The model under review builds one solid part; all positions refer to its coordinate system, in mm. Face numbers are marked on the shaded views. A direction names the side the tool comes from. Give positions to 0.01 mm unless a question says otherwise; leave off trailing zeros. Order: outer loops, then holes, each group sorted by start corner. A loop starts at its lowest first (then second) coordinate and runs counter-clockwise, first axis right, second up. Notation, with made-up numbers: (39, 5) - (71, 5) arc R6 ccw to (71, 9) - close; hole circle Ø6 at (41, 50.25). An arc over 180 degrees is marked (long way). Use CSV: the item, a comma, the result in double quotes.
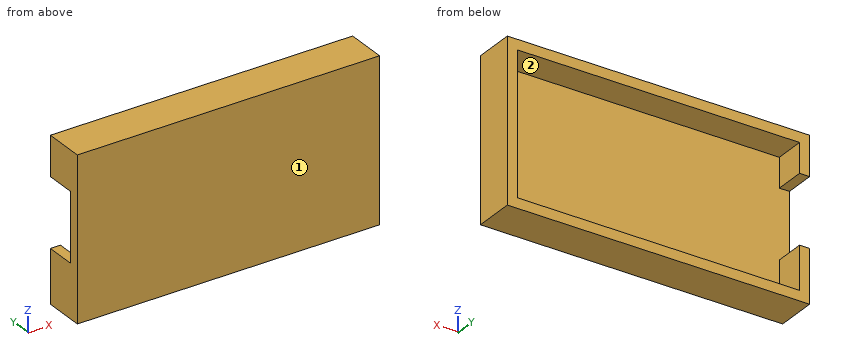
```python
from build123d import *

# Parameters (mm, degrees)
F0_W     = 2.5
F0_H     = 17
F1_DEPTH = 10
F2_DEPTH = 7.5


# Not quite as in the source:
# - a feature names something its author has since deleted; it is built from what else it names


with BuildPart() as f1:
    # F0 (on Front) → F1 (new body)
    with BuildSketch(Plane.XZ):
        Polygon((37.5, 20), (-37.5, 20), (-37.5, 10.2), (-35, 10.2), (-35, 17.5), (35, 17.5), (35, -17.5), (-35, -17.5), (-35, -6.8), (-37.5, -6.8), (-37.5, -20), (37.5, -20), align=None)
        with Locations((-36.25, 1.7)):
            Rectangle(F0_W, F0_H)
        Polygon((-35, 17.5), (-35, 10.2), (-35, -6.8), (-35, -17.5), (35, -17.5), (35, 17.5), align=None)
    extrude(amount=F1_DEPTH)

    # F0 (on Front) → F2 (cut)
    with BuildSketch(Plane.XZ):
        Polygon((-35, 17.5), (-35, 10.2), (-35, -6.8), (-35, -17.5), (35, -17.5), (35, 17.5), align=None)
        with Locations((-36.25, 1.7)):
            Rectangle(F0_W, F0_H)
    extrude(amount=F2_DEPTH, mode=Mode.SUBTRACT)


solid = f1.part
```
Item 1: Tool access review of the marked faces 1 and 2: name each direction out of +Z, -Z, +X, -X, +Y, -Y from which nothing blocks a thin tool from reaching the whole face with its end or side.
Results list:
face 1,"+Z, -Z, +X, -X, -Y"
face 2,"+Y"
Item 2: Take a section at A-A, the plane z = -12. Give the boundary of the cut face in (x, y), and give its area (3 significant figures).
Results list:
outline,"(-37.5, -10) - (37.5, -10) - (37.5, 0) - (35, 0) - (35, -7.5) - (-35, -7.5) - (-35, 0) - (-37.5, 0) - close"
area,"225 mm2"
Item 3: Take a section at D-D, the plane z = 8.5. Give the boundary of the cut face in (x, y), and give its area (3 significant figures).
Results list:
outline,"(-37.5, -10) - (37.5, -10) - (37.5, 0) - (35, 0) - (35, -7.5) - (-37.5, -7.5) - close"
area,"206 mm2"
Item 4: Take a section at C-C, the plane y = -5.75. Give the boundary of the cut face in (x, z), and give its area (4 significant figures).
Results list:
outline,"(-37.5, -20) - (37.5, -20) - (37.5, 20) - (-37.5, 20) - (-37.5, 10.2) - (-35, 10.2) - (-35, 17.5) - (35, 17.5) - (35, -17.5) - (-35, -17.5) - (-35, -6.8) - (-37.5, -6.8) - close"
area,"507.5 mm2"
Item 5: Take a section at B-B, the plane x = 29. Give the boundary of the cut face in (y, z).
Results list:
outline,"(-10, -20) - (0, -20) - (0, -17.5) - (-7.5, -17.5) - (-7.5, 17.5) - (0, 17.5) - (0, 20) - (-10, 20) - close"
Item 6: Clearance check with a flat-ended pin moving along its axis: pin 1 (6 mm diameter, centred on x = -25, z = 9, fed in from +Y). State where the tip first meets the part, or that it passes through.
Results list:
pin 1,"stops at y = -7.5"
Item 7: Wall thickness on L1, parallel to X at y = -5.5, z = -13; L2, parallel to Z at x = -27.5, y = -3.75; L3, parallel to Y at x = -5.5, z = 9: over which ranges is each line inside the solid? List them lowest first.
Results list:
L1,"x = -37.5 to -35, 35 to 37.5"
L2,"z = -20 to -17.5, 17.5 to 20"
L3,"y = -10 to -7.5"
